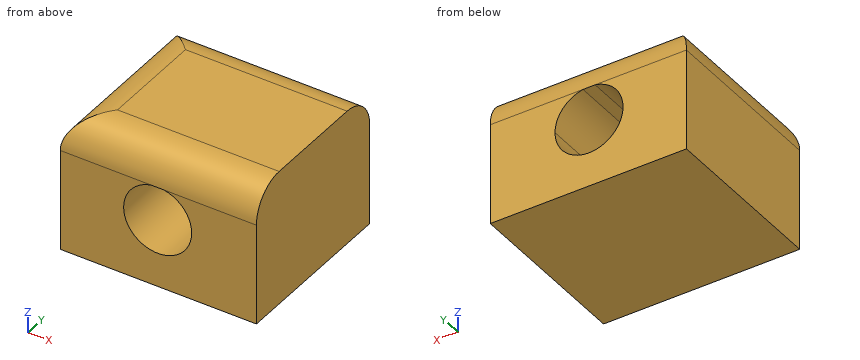
from build123d import *

# Parameters (mm, degrees)
F0_W     = 28.8251918835
F0_H     = 20
F1_DEPTH = 25.4
F2_R     = 5.08
F4_DEPTH = 25.401


with BuildPart() as f1:
    # F0 (on Front) → F1 (new body)
    with BuildSketch(Plane.XZ):
        Rectangle(F0_W, F0_H)
    extrude(amount=F1_DEPTH)

    # F2
    f2_edges = [f1.edges().sort_by_distance(p)[0] for p in [
        (0, 0, 10),
        (-14.412596, -12.7, 10),
        (0, -25.4, 10),
    ]]
    fillet(f2_edges, radius=F2_R)

    # F3 (on face) → F4 (cut, through all)
    with BuildSketch(Plane.XZ.offset(25.4)):
        with BuildLine():
            ThreePointArc((-0.9913088891, 4.92), (-3.3056021973, -3.8375911383), (4.899533409, 0))
            ThreePointArc((4.899533409, 0), (3.7371245473, 3.2051356063), (0.790375707, 4.92))
            Line((0.790375707, 4.92), (-0.9913088891, 4.92))
        make_face()
    extrude(amount=-F4_DEPTH, mode=Mode.SUBTRACT)


solid = f1.part
Could you check a few things on this model? Use its own coordinates, in mm. Coordinates: 2 decimals unless noted, no trailing zeros. Write each loop counter-clockwise with the first axis right and the second up, starting at its lowest first coordinate (ties: lowest second). Pieces come first, ordered by that corner, then holes. Notation, with made-up numbers: (48, 70.25) - (97, 70.25) arc R19 ccw to (97, 96.25) - close; hole circle Ø10 at (29, 70). An arc over 180 degrees is marked (long way). Put each result on its own line as item: value. Start each with the question number.
Q1. I want a section at C-C on x = -7.75. Write out the boundary of the cut face in (y, z).
Q2. Please list where these lines run through material, in increasing order: L1, parallel to X at y = -18, z = 0; L2, parallel to X at y = -24, z = -1.75; L3, parallel to Z at x = -3.5, y = -5.
Q3. I want a section at A-A on y = -8. Write out the boundary of the cut face in (x, z).
Q4. I want a section at B-B on x = -3.25. Write out the boundary of the cut face in (y, z), plus the area to 3 significant figures.
Q5. I want a section at D-D on y = -20.75. Write out the boundary of the cut face in (x, z).
Q6. I'm going to push flat-ended pins straight in: P1, Ø12, axis at x = -5, z = 6.5, coming from the +Y side; P2, Ø4, axis at x = 1, z = 1.5, coming from the -Y side. Where does each tip first touch, or does it pass through?
Checks:
1. outline: (-25.4, -10) - (0, -10) - (0, 4.92) arc R5.08 ccw to (-5.08, 10) - (-20.32, 10) arc R5.08 ccw to (-25.4, 4.92) - close
2. L1: -14.41 to -5.1, 4.9 to 14.41
2. L2: -14.41 to -4.78, 4.58 to 14.41
2. L3: -10 to -3.67, 3.67 to 10
3. outline: (-14.41, -10) - (14.41, -10) - (14.41, 10) - (-9.33, 10) arc R5.08 ccw to (-14.41, 4.92) - close; hole (-0.99, 4.92) arc R5 ccw (long way) to (0.79, 4.92) - close
4. outline: (-25.4, -10) - (0, -10) - (0, -3.88) - (-25.4, -3.88) - close; (-25.4, 3.88) - (0, 3.88) - (0, 4.92) arc R5.08 ccw to (-5.08, 10) - (-20.32, 10) arc R5.08 ccw to (-25.4, 4.92) - close
4. area: 300 mm²
5. outline: (-14.41, -10) - (14.41, -10) - (14.41, 9.98) - (-9.76, 9.98) arc R5.08 ccw to (-14.41, 4.92) - close; hole (-0.99, 4.92) arc R5 ccw (long way) to (0.79, 4.92) - close
6. P1: y = 0
6. P2: through
